The drawing under review shows one solid part. Ordinate dimensions are in mm from its lowest x, y, z. A direction names the side the tool comes from. Give positions to 0.01 mm unless a question says otherwise; leave off trailing zeros. Order: outer loops, then holes, each group sorted by start corner. A loop starts at its lowest first (then second) coordinate and runs counter-clockwise, first axis right, second up. Notation, with made-up numbers: (-15, 52.25) -> (-11, 52.25) arc R29 cw to (-11, 85.25) -> close; hole circle Ø1 at (-24.75, 7.5). An arc over 180 degrees is marked (long way). Return JSON: item names as keys, results as strings. Group by question number.
1) For the marked faces 1, 2 and 3, list the 3-axis set-ups (+Z, -Z, +X, -X, +Y, -Y) from which the entire face can be reached by the end or side of a thin tool; tool diameter is ignored.
2) Insertion check: P1, Ø3, axis at y = 28, z = 4.5, coming from the +X side; P2, Ø5, axis at y = 22.5, z = 7, coming from the -X side; P3, Ø5, axis at x = 9.5, z = 5, coming from the -Y side; P4, Ø12, axis at x = 10.5, y = 31.5, coming from the -Z side. Each pin has a flat end and moves straight along its axis. Give the tip position at first contact, or say it passes through.
3) Add section C-C (y = 24). Give the boundary of the cut face in (x, z).
4) Add section A-A (z = 11.25). Give the boundary of the cut face in (x, y).
5) Add section B-B (x = 30). Give the boundary of the cut face in (y, z).
6) The part is to be moulded in two halves that separate along X. For the marked faces 4, 5 and 6, say which applies: released by +X, released by -X, zero draft, split by the parting line, or undercut.
7) To check wall thickness, follow line 1 along Y through (x, z) = (9, 11); line 2 along X through (y, z) = (22.5, 3.5); line 3 along X through (y, z) = (34.4, 7). State the ranges of each line that lie inside material, in increasing order.
8) Add section D-D (z = 7). Give the boundary of the cut face in (x, y), then the cut area to 3 significant figures.
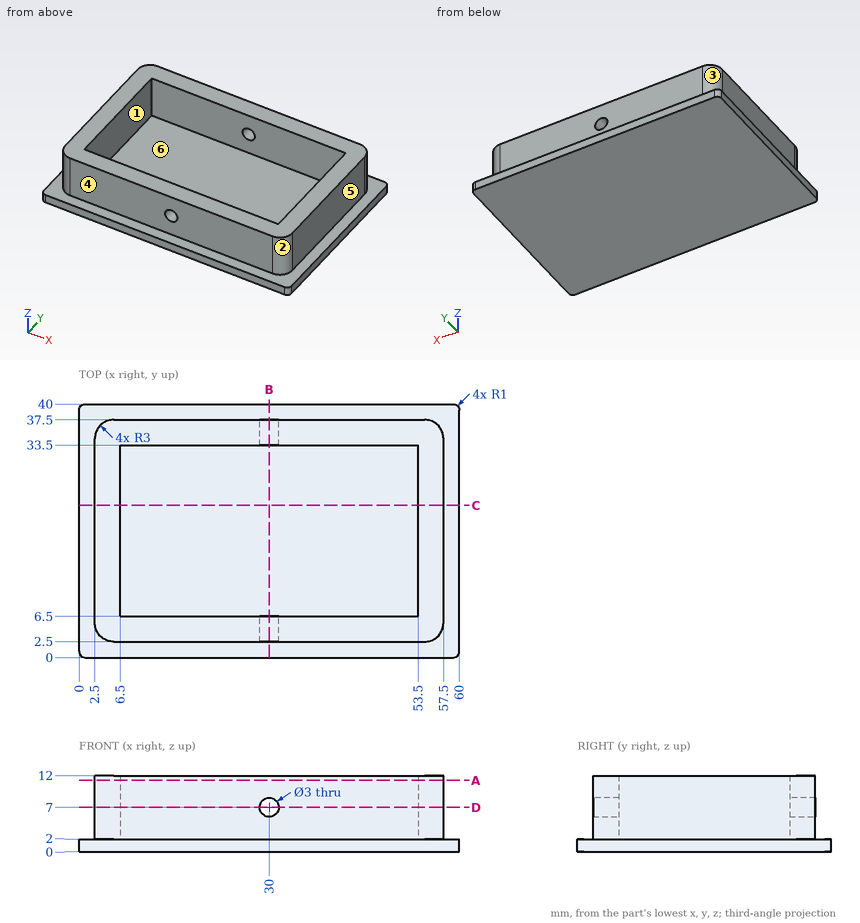
Evaluation:
{
 "1": {"face 1": "+Z", "face 2": "+Z, +X, -Y", "face 3": "+Z, -X, +Y"},
 "2": {"P1": "x = 57.5", "P2": "x = 2.5", "P3": "y = 2.5", "P4": "z = 0"},
 "3": {"outline": "(0, 0) -> (60, 0) -> (60, 2) -> (57.5, 2) -> (57.5, 12) -> (53.5, 12) -> (53.5, 2) -> (6.5, 2) -> (6.5, 12) -> (2.5, 12) -> (2.5, 2) -> (0, 2) -> close"},
 "4": {"outline": "(2.5, 5.5) arc R3 ccw to (5.5, 2.5) -> (54.5, 2.5) arc R3 ccw to (57.5, 5.5) -> (57.5, 34.5) arc R3 ccw to (54.5, 37.5) -> (5.5, 37.5) arc R3 ccw to (2.5, 34.5) -> close; hole (6.5, 6.5) -> (53.5, 6.5) -> (53.5, 33.5) -> (6.5, 33.5) -> close"},
 "5": {"outline": "(0, 0) -> (40, 0) -> (40, 2) -> (37.5, 2) -> (37.5, 5.5) -> (33.5, 5.5) -> (33.5, 2) -> (6.5, 2) -> (6.5, 5.5) -> (2.5, 5.5) -> (2.5, 2) -> (0, 2) -> close; (2.5, 8.5) -> (6.5, 8.5) -> (6.5, 12) -> (2.5, 12) -> close; (33.5, 8.5) -> (37.5, 8.5) -> (37.5, 12) -> (33.5, 12) -> close"},
 "6": {"face 4": "zero draft", "face 5": "released by +X", "face 6": "undercut"},
 "7": {"line 1": "2.5 to 6.5, 33.5 to 37.5", "line 2": "2.5 to 6.5, 53.5 to 57.5", "line 3": "2.5 to 28.5, 31.5 to 57.5"},
 "8": {"outline": "(2.5, 5.5) arc R3 ccw to (5.5, 2.5) -> (28.5, 2.5) -> (28.5, 6.5) -> (6.5, 6.5) -> (6.5, 33.5) -> (28.5, 33.5) -> (28.5, 37.5) -> (5.5, 37.5) arc R3 ccw to (2.5, 34.5) -> close; (31.5, 2.5) -> (54.5, 2.5) arc R3 ccw to (57.5, 5.5) -> (57.5, 34.5) arc R3 ccw to (54.5, 37.5) -> (31.5, 37.5) -> (31.5, 33.5) -> (53.5, 33.5) -> (53.5, 6.5) -> (31.5, 6.5) -> close", "area": "624 mm^2"}
}
